```python
from build123d import *

# Parameters (mm, degrees)
SKETCH3_R               = 3.175
BOSS_EXTRUDE1_DEPTH     = 304.8
CHAMFER1_SIZE           = 0.635
CUT_EXTRUDE1_START      = -93.519625
SKETCH4_R               = 3.175
CUT_EXTRUDE1_DEPTH      = 517.080375
SKETCH5_R               = 0.5953125
CUT_EXTRUDE2_DEPTH      = 4.175
CUT_EXTRUDE2_DEPTH_BACK = 4.175


with BuildPart() as part:
    # Sketch3 → Boss-Extrude1 (new body, symmetric)
    with BuildSketch(Plane.XY):
        Circle(SKETCH3_R)
    extrude(amount=BOSS_EXTRUDE1_DEPTH, both=True)

    # Chamfer1
    chamfer1_edges = [part.edges().sort_by_distance(p)[0] for p in [
        (-3.175, 0, -304.8),
        (-3.175, 0, 304.8),
    ]]
    chamfer(chamfer1_edges, length=CHAMFER1_SIZE)

    # Sketch4 → Cut-Extrude1 (cut, through all)
    with BuildSketch(Plane.XY.offset(304.8).offset(CUT_EXTRUDE1_START)):
        Circle(SKETCH4_R)
    extrude(amount=-CUT_EXTRUDE1_DEPTH, mode=Mode.SUBTRACT)

    # Sketch5 → Cut-Extrude2 (cut, two sides)
    with BuildSketch(Plane(origin=(0, 0, 0), x_dir=(1, 0, 0), z_dir=(0, 1, 0))) as cut_extrude2_sk:
        with Locations((0, -212.867875)):
            Circle(SKETCH5_R)
        with Locations((0, -303.2125)):
            Circle(SKETCH5_R)
    extrude(amount=CUT_EXTRUDE2_DEPTH, mode=Mode.SUBTRACT)
    extrude(cut_extrude2_sk.sketch, amount=-CUT_EXTRUDE2_DEPTH_BACK, mode=Mode.SUBTRACT)


solid = part.part
```
Geometry: final body of the model. Coordinates: model frame, mm. Coordinates: 2 decimals unless noted, no trailing zeros. Write each loop counter-clockwise with the first axis right and the second up, starting at its lowest first coordinate (ties: lowest second). Pieces come first, ordered by that corner, then holes. Notation, with made-up numbers: M 2,49.5 L 61,49.5 A30 cw 61,79.5 Z; hole C 17.5,9.25 d2. An arc over 180 degrees is marked long. Use CSV: the item, a comma, the result in double quotes. Start each with the question number.
1. Ray query, probe 1 along Z at (x, y) = (0, 0.95); probe 2 along Z at (x, y) = (0.5, -1.25); probe 3 along X at (y, z) = (0.25, 294). Return the intervals inside material, ascending.
2. Cut plane B-B on z = 286.5. Return the cut outline in (x, y) (3 decimals).
3. Cut plane A-A on y = -1.5. Count the separate pieces of the cut face and the enclosed holes in it, plus the area to 3 significant figures.
4. First-contact query: P1, Ø1, axis at y = 2, z = 292.5, coming from the +X side. Flat tip, straight axial feed; report the tip coordinate or a pass-through.
Entries:
1,probe 1,"211.28 to 212.27, 213.46 to 302.62, 303.81 to 304.8"
1,probe 2,"211.28 to 212.54, 213.19 to 302.89, 303.54 to 304.8"
1,probe 3,"-3.17 to 3.17"
2,outline,"C 0,0 d6.35"
3,separate pieces,"1"
3,enclosed holes,"2"
3,area,"521 mm²"
4,P1,"x = 2.8"
